from build123d import *

# Parameters (mm, degrees)
F0_W     = 199.3581205606
F0_H     = 119.528003037
F1_DEPTH = 127
F2_R     = 6.35
F3_T     = -2.54


# Not quite as in the source:
# - a shell that OpenCascade refuses in one call is made with other operations: the cavity is built on its own and cut out


with BuildPart() as f1:
    # F0 (on Top) → F1 (new body)
    with BuildSketch(Plane.XY):
        with Locations((-20.9509953856, 1.4819204807)):
            Rectangle(F0_W, F0_H)
    extrude(amount=F1_DEPTH)

    # F2
    f2_edges = [f1.edges().sort_by_distance(p)[0] for p in [
        (-20.950995, -58.282081, 127),
        (78.728065, 1.48192, 127),
        (-20.950995, 61.245922, 127),
        (-120.630056, 1.48192, 127),
        (-120.630056, -58.282081, 63.5),
        (78.728065, -58.282081, 63.5),
    ]]
    fillet(f2_edges, radius=F2_R)

    # F3: a shell. OpenCascade refuses it in one call, so the cavity is built on its own and cut out:
    # the body offset inwards by the wall thickness, plus a prism from it out through each open face.
    f3_core = offset(f1.part, amount=F3_T, mode=Mode.PRIVATE)
    f3_exits = [f3_core.faces().sort_by_distance(p)[0] for p in [
        (-20.950995, -55.742081, 61.595),
    ]]
    add(f3_core, mode=Mode.SUBTRACT)
    extrude(f3_exits, amount=-F3_T, mode=Mode.SUBTRACT)


solid = f1.part
Model file for the job. Use its own axes, mm. A direction names the side the tool comes from. Give positions to 0.01 mm unless a question says otherwise; leave off trailing zeros. Order: outer loops, then holes, each group sorted by start corner. A loop starts at its lowest first (then second) coordinate and runs counter-clockwise, first axis right, second up. Notation, with made-up numbers: (-17.75, 75) - (6.25, 75) arc R20 ccw to (6.25, 93) - close; hole circle Ø4 at (19, -25.75). An arc over 180 degrees is marked (long way). Return JSON: item names as keys, results as strings.
1) Cut at B-B, the plane x = 56. Give the cut face in (y, z), plus the area to 3 significant figures.
Geometry says:
{"outline": "(-58.28, 0) - (61.25, 0) - (61.25, 120.65) arc R6.35 ccw to (54.9, 127) - (-51.93, 127) arc R6.35 ccw to (-58.28, 120.65) - (-55.74, 120.65) arc R3.81 cw to (-51.93, 124.46) - (54.9, 124.46) arc R3.81 cw to (58.71, 120.65) - (58.71, 2.54) - (-58.28, 2.54) - close", "area": "915 mm²"}
2) Cut at C-C, the plane z = 110. Give the cut face in (x, y), plus the area to 3 significant figures.
Geometry says:
{"outline": "(-120.63, -51.93) arc R6.35 ccw to (-114.28, -58.28) - (-114.28, -55.74) arc R3.81 cw to (-118.09, -51.93) - (-118.09, 58.71) - (76.19, 58.71) - (76.19, -51.93) arc R3.81 cw to (72.38, -55.74) - (72.38, -58.28) arc R6.35 ccw to (78.73, -51.93) - (78.73, 61.25) - (-120.63, 61.25) - close", "area": "1,110 mm²"}
3) Pull direction Z, two halves, no side cores. Call faces 3 (the flat face through (-22, 2, 124.46)), 4 (the cylindrical face through (76.82, -56.47, 61.17)), 5 (the flat face through (-22, 2, 0)), 6 (the cylindrical face through (76.92, 5.45, 125.09)): pulls with the +Z half, pulls with the -Z half, needs draft (parallel to the pull), parting line crosses it, or undercut.
Geometry says:
{"face 3": "undercut", "face 4": "needs draft", "face 5": "pulls with the -Z half", "face 6": "pulls with the +Z half"}
4) 3-axis set-ups, long thin cutter, end or side, ignore diameter. For faces 1 (the cylindrical face through (-118.82, 5.45, 125.09)), 2 (the flat face through (76.188, 3, 61)): which of +Z, -Z, +X, -X, +Y, -Y reach the whole face in a straight line?
Geometry says:
{"face 1": "+Z, -X, +Y, -Y", "face 2": "none"}
5) Cut at A-A, the plane y = -15.5. Give the cut face in (x, z).
Geometry says:
{"outline": "(-120.63, 0) - (78.73, 0) - (78.73, 120.65) arc R6.35 ccw to (72.38, 127) - (-114.28, 127) arc R6.35 ccw to (-120.63, 120.65) - close; hole (-118.09, 2.54) - (76.19, 2.54) - (76.19, 120.65) arc R3.81 ccw to (72.38, 124.46) - (-114.28, 124.46) arc R3.81 ccw to (-118.09, 120.65) - close"}
6) Probe line 1 (X direction, y = 12, z = 76); line 2 (Z direction, x = -10.5, y = 41); line 3 (Y direction, x = -18.5, z = 48.5). List the from-to ranges inside material, lowest first. Write a range as from..to.
Geometry says:
{"line 1": "-120.63..-118.09, 76.19..78.73", "line 2": "0..2.54, 124.46..127", "line 3": "58.71..61.25"}
7) Flat gauge pins, fed straight in: P1, Ø2, axis at x = 7.5, z = 69, coming from the -Y side; P2, Ø0.8, axis at y = -57.5, z = 54, coming from the -X side; P3, Ø2, axis at y = -56.5, z = 32.5, coming from the +X side. Where does each tip first touch, or does it go through?
Geometry says:
{"P1": "y = 58.71", "P2": "x = -117.97", "P3": "x = 77.63"}
